Input: part model. Units: mm. Frame: model coordinates. A direction names the side the tool comes from. Round coordinates to 2 decimals unless told otherwise and drop trailing zeros. Order: outer loops, then holes, each group sorted by start corner. A loop starts at its lowest first (then second) coordinate and runs counter-clockwise, first axis right, second up. Notation, with made-up numbers: (-21.5, -26.75) -> (2.5, -26.75) arc R15 ccw to (2.5, -10.75) -> close; hole circle Ø10 at (4.5, 34). An arc over 180 degrees is marked (long way). Use a Markdown table: item, result.
Autodesk Inventor part; units mm, degrees
ref_plane "YZ Plane" through (0, 0, 0) normal (1, 0, 0) x (0, 1, 0)
ref_plane "XZ Plane" through (0, 0, 0) normal (0, 1, 0) x (-1, 0, 0)
ref_plane "XY Plane" through (0, 0, 0) normal (0, 0, 1) x (1, 0, 0)
sketch "Эскиз1" plane through (0, 0, 0) normal (0, 0, 1) x (1, 0, 0)
  line L0 (0, 30) -> (-120, 30)
  line L1 (-120, 30) -> (-120, 6)
  line L2 (-120, 6) -> (-75, 6)
  line L3 (-75, 6) -> (-75, 0)
  line L4 (-75, 0) -> (-51, 0)
  line L5 (-51, 0) -> (-51, 15)
  line L6 (-51, 15) -> (-34, 15)
  line L7 (-34, 15) -> (-34, 30)
  line L8 (0, 0) -> (0, 30)
  dimension "d31" = 120
  dimension "d32" = 24
  dimension "d33" = 45
  dimension "d34" = 24
  dimension "d35" = 15
  dimension "d36" = 17
  dimension "d38" = 30
revolve "Вращение1" add sketch "Эскиз1" angle 360 about axis through (0, 0, 0) along (0, 1, 0)
sketch "Эскиз2" plane through (0, 30, 0) normal (0, 1, 0) x (1, 0, 0)
  line L0 (0, 0) -> (0, 107.5)
  dimension "d37" = 107.5
hole "Отверстие1" at (0, 30, -107.5) direction (0, -1, 0) diameter 14 end through all
pattern_circular "Круговой массив2" count 8 over 360 about axis through (0, 18, 0) along (0, -1, 0) of "Отверстие1"
sketch "Эскиз3" plane through (0, 30, 0) normal (0, 1, 0) x (1, 0, 0)
  line L0 (0, 0) -> (67, 0)
  circle A0 centre (67, 0) radius 2
  dimension "d39" = 67
  dimension "d40" = 4
extrude "Выдавливание1" cut sketch "Эскиз3" against normal through all
sketch "Эскиз4" plane through (0, 30, 0) normal (0, 1, 0) x (1, 0, 0)
  circle A0 centre (67, 0) radius 2
  point P0 (0, 0)
hole "Отверстие2" at (67, 30, 0) direction (0, -1, 0) diameter 12 depth 13 tip angle 118 counterbore diameter 14 counterbore depth 11.25
thread "Резьба1"
pattern_circular "Круговой массив3" count 2 over 360 about axis through (0, 22.5, 0) along (0, -1, 0) of "Отверстие2", "Выдавливание1"
sketch "Эскиз8" plane through (0, 30, 0) normal (0, 1, 0) x (1, 0, 0)
  line L0 (0, 0) -> (0, 64)
  circle A0 centre (0, 64) radius 4
  dimension "d66" = 64
  dimension "d67" = 8
extrude "Выдавливание3" cut sketch "Эскиз8" against normal through all
sketch "Эскиз9" plane through (0, 30, 0) normal (0, 1, 0) x (1, 0, 0)
  circle A0 centre (0, 64) radius 4
  point P0 (0, 0)
hole "Отверстие3" at (0, 30, -64) direction (0, -1, 0) diameter 12 depth 13 tip angle 118 counterbore diameter 14 counterbore depth 11.25
thread "Резьба2"
pattern_circular "Круговой массив4" count 2 over 360 about axis through (0, 22.5, 0) along (0, -1, 0) of "Отверстие3", "Выдавливание3"
sketch "Эскиз11" plane through (0, 30, 0) normal (0, 1, 0) x (1, 0, 0)
  circle A0 centre (49.7929, 41.7812) radius 1.5
  circle A1 centre (56.2917, -32.5) radius 1.5
  circle A2 centre (-64.0125, -11.2871) radius 1.5
  point P0 (0, 0)
extrude "Выдавливание5" cut sketch "Эскиз11" against normal blind 40
properties part number "Крышка сальников" material "Чугун, серый"
1) Cut plane B-B on z = 21. Return loops of the section in (x, y).
Results found:
| item | result |
|---|---|
| outline | (-118.15, 6) -> (-72, 6) -> (-72, 0) -> (-46.48, 0) -> (-46.48, 15) -> (-26.74, 15) -> (-26.74, 30) -> (-118.15, 30) -> close; (26.74, 15) -> (46.48, 15) -> (46.48, 0) -> (72, 0) -> (72, 6) -> (118.15, 6) -> (118.15, 30) -> (26.74, 30) -> close |
2) Pull-direction query (Z, two-part tool) for faces 1 (the flat face through (65, 18.75, 6)), 2 (the flat face through (-25, 30, -25)), 3 (the cylindrical face through (119.884, 17.832, -5.276)); classes: +Z half, -Z half, draft (parallel to the pull), parting line (faces both ways), or undercut.
Results found:
| item | result |
|---|---|
| face 1 | undercut |
| face 2 | draft |
| face 3 | parting line |
3) Pin query (flat end, axial travel): pin 1 Ø7 at (x, z) = (67, 0) entering from +Y; pin 2 Ø3 at (y, z) = (14, 66.5) entering from +X; pin 3 Ø6 at (y, z) = (12, -80.5) entering from +X. Return the tip coordinate at first contact, or that it passes through.
Results found:
| item | result |
|---|---|
| pin 1 | stops at y = 15.5 |
| pin 2 | stops at x = 100.87 |
| pin 3 | stops at x = 91.62 |
4) Set-up query: faces 4 (the cylindrical face through (2.103, 24.296, 57.323)), 5 (the flat face through (-33, 15, -11)), 6 (the cylindrical face through (0.867, 8.01, 60.095)). Return all of +Z, -Z, +X, -X, +Y, -Y with unobstructed straight access to the full face (end or side cutting, diameter ignored); none if empty.
Results found:
| item | result |
|---|---|
| face 4 | +Y |
| face 5 | -Y |
| face 6 | +Y, -Y |
5) Cut plane D-D on z = 64. Return loops of the section in (x, y).
Results found:
| item | result |
|---|---|
| outline | (-101.51, 6) -> (-39.1, 6) -> (-39.1, 0) -> (-4, 0) -> (-4, 15.8) -> (-6, 17) -> (-6, 18.75) -> (-7, 18.75) -> (-7, 30) -> (-101.51, 30) -> close; (4, 0) -> (39.1, 0) -> (39.1, 6) -> (101.51, 6) -> (101.51, 30) -> (7, 30) -> (7, 18.75) -> (6, 18.75) -> (6, 17) -> (4, 15.8) -> close |
6) Cut plane C-C on y = 22. Count the separate pieces of the cut face and the enclosed holes in it, and give its area (3 significant figures).
Results found:
| item | result |
|---|---|
| separate pieces | 1 |
| enclosed holes | 16 |
| area | 39,700 mm² |
7) Cut plane A-A on x = 10.5. Return loops of the section in (y, z), and give its area (3 significant figures).
Results found:
| item | result |
|---|---|
| outline | (0, -74.26) -> (6, -74.26) -> (6, -119.54) -> (30, -119.54) -> (30, -32.34) -> (15, -32.34) -> (15, -49.91) -> (0, -49.91) -> close; (0, 49.91) -> (15, 49.91) -> (15, 32.34) -> (30, 32.34) -> (30, 119.54) -> (6, 119.54) -> (6, 74.26) -> (0, 74.26) -> close |
| area | 4,160 mm² |
8) Line query: L1, parallel to Y at x = 46.5, z = -83.5; L2, parallel to X at y = 14, z = -107.5; L3, parallel to Z at x = -2.5, y = 7. Output: solid intervals per line, ascending. Write a range as [from, to].
Results found:
| item | result |
|---|---|
| L1 | y = [6, 30] |
| L2 | x = [-53.33, -7], [7, 53.33] |
| L3 | z = [-119.97, -114.04], [-100.96, -67.12], [-60.88, -50.94], [50.94, 60.88], [67.12, 100.96], [114.04, 119.97] |
